Work out the finished part from the listing and answer in its coordinate system (mm). A direction names the side the tool comes from. Give positions to 0.01 mm unless a question says otherwise; leave off trailing zeros. Loops run counter-clockwise (first coordinate to the right, second up) from the corner with the lowest first, then second, coordinate; pieces in that order, holes last. Notation, with made-up numbers: (41.5, -23.75) - (53.5, -23.75) arc R11 cw to (53.5, -11.75) - close; hole circle Ø3 at (69.5, -37). An arc over 180 degrees is marked (long way). One line per question, with ' | ' between items. Start each with the question number.
1. Section B-B (y = -22.5) is taken. Determine the outline of the cut face in (x, z), plus the area to 3 significant figures.
2. Find the intervals of material crossed by line 1 (X direction, y = -39.5, z = 29.5); line 2 (Z direction, x = -25, y = -47.5); line 3 (Y direction, x = -34, z = 11), in increasing order.
3. Which of the six approach directions +Z, -Z, +X, -X, +Y, -Y give full straight-line access (tool end or side, diameter ignored) to faces 4 (the face through (-34.49, -24.89, 13.21)), 5 (the face through (3, -28, 31.506))?
4. For a pull along X with two mould halves and no side action, classify faces 1 (the face through (20.929, -33.456, 36.336)), 2 (the face through (-32, 0, 20)), 3 (the face through (-29.662, -28, -2)) as released by +X, released by -X, zero draft, split by the parting line, or undercut.
5. Section A-A (z = 8.5) is taken. Determine the outline of the cut face in (x, y).
6. Section D-D (x = 14.5) is taken. Determine the outline of the cut face in (y, z).
7. Each of these flat-tipped pins is pushed along its axis until it touches: pin 1 (4 mm diameter, centred on x = 0.5, y = -8, fed in from -Z); pin 2 (8 mm diameter, centred on y = -39, z = 9, fed in from +X); pin 3 (6 mm diameter, centred on y = -28.58, z = -20.17, fed in from -X). Where does it stop, or does it pass through?
8. Section C-C (x = -33.5) is taken. Determine the outline of the cut face in (y, z) (3 decimals).
from build123d import *

# Parameters (mm, degrees)
F1_DEPTH = 57.15
F3_R     = 5
F4_DEPTH = 25
F2_R     = 5
F5_DEPTH = 25


with BuildPart() as f1:
    # F0 (on Front) → F1 (new body)
    with BuildSketch(Plane.XZ):
        Polygon((37.012778, 41.031351), (-39.187222, 41.031351), (-39.187222, -35.168649), (-29.662222, -35.168649), (-29.662222, 31.506351), (37.012778, 31.506351), align=None)
    extrude(amount=F1_DEPTH)

    # F3 (on face) → F4 (cut)
    with BuildSketch(Plane(origin=(-39.187222, 0, 0), x_dir=(0, -1, 0), z_dir=(-1, 0, 0))):
        with Locations((28.575, -20.168649)):
            Circle(F3_R)
        with Locations((28.575, 9.831351)):
            Circle(F3_R)
    extrude(amount=-F4_DEPTH, mode=Mode.SUBTRACT)

    # F2 (on face) → F5 (cut)
    with BuildSketch(Plane.XY.offset(41.031351)):
        with Locations((-7.987222, -28.575)):
            Circle(F2_R)
        with Locations((22.012778, -28.575)):
            Circle(F2_R)
    extrude(amount=-F5_DEPTH, mode=Mode.SUBTRACT)


solid = f1.part
Conclusion:
1) outline: (-39.19, -35.17) - (-29.66, -35.17) - (-29.66, 31.51) - (37.01, 31.51) - (37.01, 41.03) - (-39.19, 41.03) - close | area: 1,360 mm²
2) line 1: -39.19 to -29.66 | line 2: 31.51 to 41.03 | line 3: -57.15 to -33.44, -23.71 to 0
3) face 4: +X, -X | face 5: -Z, +X, +Y, -Y
4) face 1: undercut | face 2: zero draft | face 3: released by +X
5) outline: (-39.19, -57.15) - (-29.66, -57.15) - (-29.66, -33.39) - (-39.19, -33.39) - close; (-39.19, -23.76) - (-29.66, -23.76) - (-29.66, 0) - (-39.19, 0) - close
6) outline: (-57.15, 31.51) - (0, 31.51) - (0, 41.03) - (-57.15, 41.03) - close
7) pin 1: z = 31.51 | pin 2: x = -29.66 | pin 3: through
8) outline: (-57.15, -35.169) - (0, -35.169) - (0, 41.031) - (-57.15, 41.031) - close; hole circle Ø10 at (-28.575, -20.169); hole circle Ø10 at (-28.575, 9.831)
